Geometry check sheet. Reference: drawing and pictorial views, mm from the part's lowest x, y, z. A direction names the side the tool comes from. Give positions to 0.01 mm unless a question says otherwise; leave off trailing zeros. Loops run counter-clockwise (first coordinate to the right, second up) from the corner with the lowest first, then second, coordinate; pieces in that order, holes last. Notation, with made-up numbers: (61, 15) - (115, 15) arc R16 cw to (115, 19) - close; hole circle Ø8 at (-21, -30.5). An arc over 180 degrees is marked (long way). Use CSV: the item, a comma, the result in double quotes.
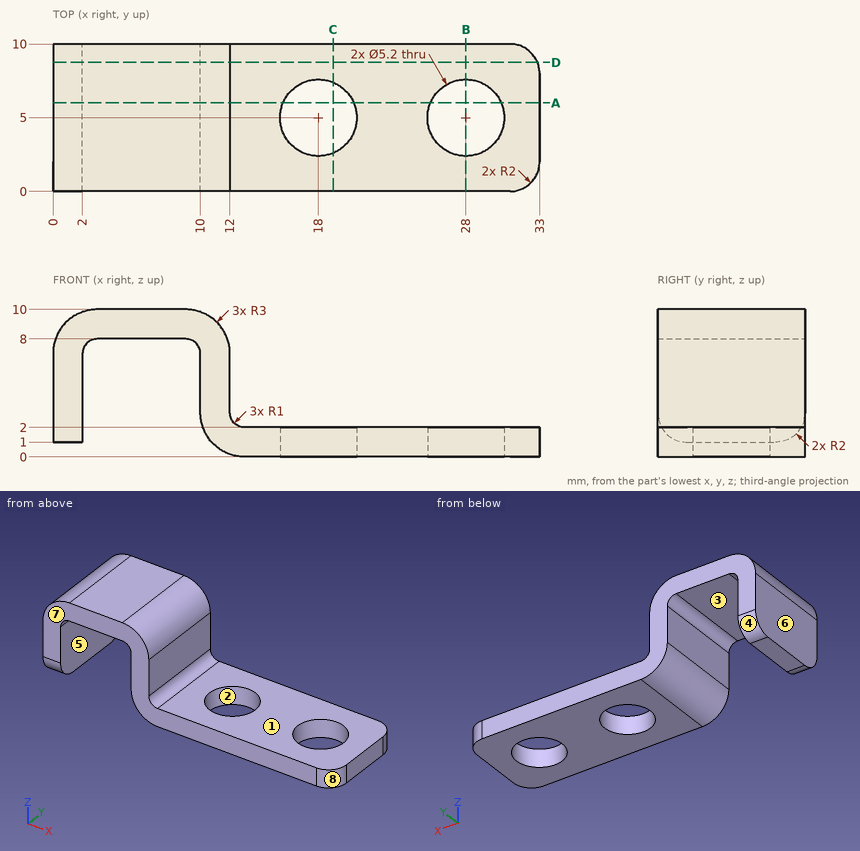
1. Scan lines: line 1 along Y through (x, z) = (18, 0.9); line 2 along X through (y, z) = (2, 3.5); line 3 along Z through (x, y) = (18.5, 1.5). Record each from-to range of solid material in increasing order.
Completed:
line 1,"y = 0 to 2.4, 7.6 to 10"
line 2,"x = 0 to 2, 10 to 12"
line 3,"z = 0 to 2"
2. Sectioned sample at C-C, the plane x = 19. Record the boundary of the cut face in (y, z), and give its area (3 significant figures).
Completed:
outline,"(0, 0) - (2.6, 0) - (2.6, 2) - (0, 2) - close; (7.4, 0) - (10, 0) - (10, 2) - (7.4, 2) - close"
area,"10.4 mm²"
3. Release check for a two-part mould opening along X. For the marked faces 5, 6, 7 and 8 record: released by +X, released by -X, zero draft, split by the parting line, or undercut.
Completed:
face 5,"undercut"
face 6,"released by -X"
face 7,"zero draft"
face 8,"released by +X"
4. Sectioned sample at B-B, the plane x = 28. Record the boundary of the cut face in (y, z), and give its area (3 significant figures).
Completed:
outline,"(0, 0) - (2.4, 0) - (2.4, 2) - (0, 2) - close; (7.6, 0) - (10, 0) - (10, 2) - (7.6, 2) - close"
area,"9.60 mm²"
5. Sectioned sample at D-D, the plane y = 8.75. Record the boundary of the cut face in (x, z), and give its area (3 significant figures).
Completed:
outline,"(0, 1.15) - (2, 1.15) - (2, 7) arc R1 cw to (3, 8) - (9, 8) arc R1 cw to (10, 7) - (10, 3) arc R3 ccw to (13, 0) - (32.85, 0) - (32.85, 2) - (13, 2) arc R1 cw to (12, 3) - (12, 7) arc R3 ccw to (9, 10) - (3, 10) arc R3 ccw to (0, 7) - close"
area,"90.3 mm²"
6. Set-up check for the marked faces 1, 2, 3 and 4: record each of +Z, -Z, +X, -X, +Y, -Y from which the full face is reachable in a straight line by a thin tool's end or side.
Completed:
face 1,"+Z, +X, +Y, -Y"
face 2,"+Z, -Z"
face 3,"-Z, +Y, -Y"
face 4,"-Z, -X, +Y"
7. Sectioned sample at A-A, the plane y = 6. Record the boundary of the cut face in (x, z).
Completed:
outline,"(0, 1) - (2, 1) - (2, 7) arc R1 cw to (3, 8) - (9, 8) arc R1 cw to (10, 7) - (10, 3) arc R3 ccw to (13, 0) - (15.6, 0) - (15.6, 2) - (13, 2) arc R1 cw to (12, 3) - (12, 7) arc R3 ccw to (9, 10) - (3, 10) arc R3 ccw to (0, 7) - close; (20.4, 0) - (25.6, 0) - (25.6, 2) - (20.4, 2) - close; (30.4, 0) - (33, 0) - (33, 2) - (30.4, 2) - close"
8. Go/stop test with flat-tipped pins: pin 1 Ø1.5 at (y, z) = (1.5, 6.5) entering from +X; pin 2 Ø2 at (x, y) = (9.5, 8.5) entering from -Z; pin 3 Ø1.6 at (x, y) = (1.5, 5.5) entering from -Z; pin 4 Ø4.5 at (x, y) = (28, 5) entering from -Z. Record where each tip stops, or that it passes through.
Completed:
pin 1,"stops at x = 12"
pin 2,"stops at z = 1.34"
pin 3,"stops at z = 1"
pin 4,"passes through"
